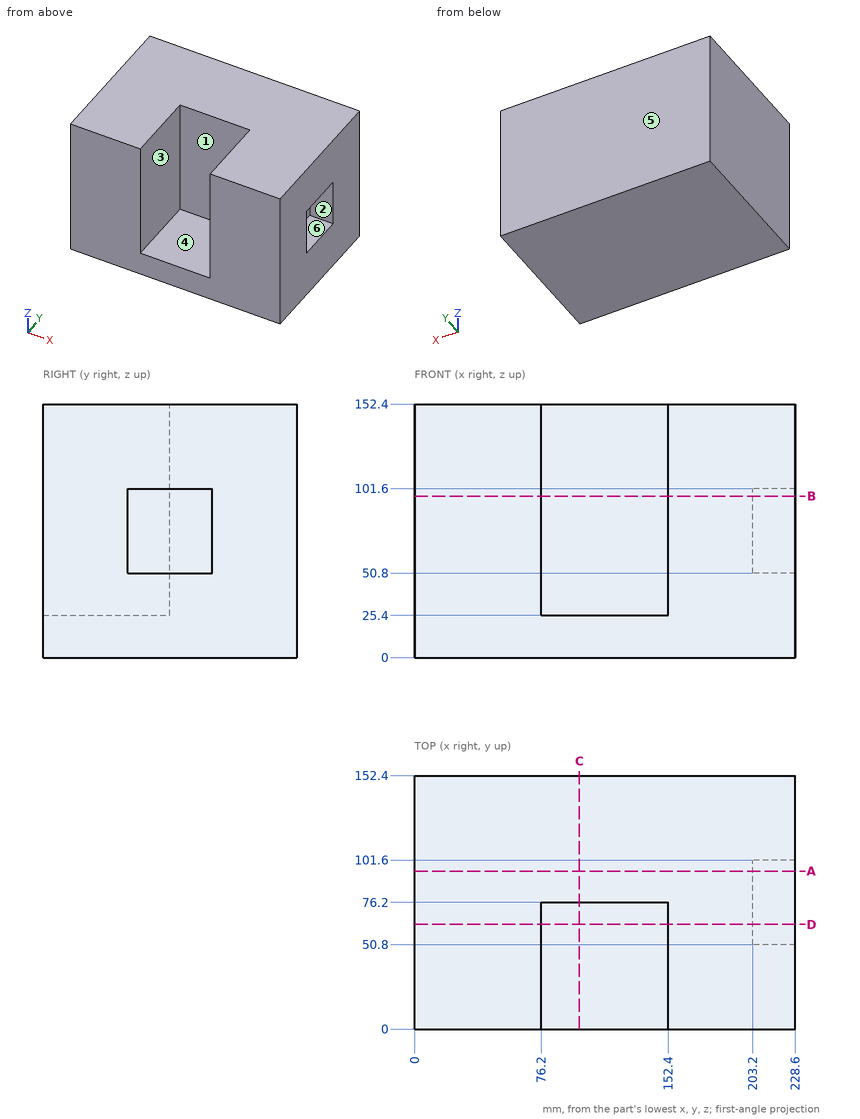
Print and shaded views of the part. All mm, measured from the part's lowest x, y and z. A direction names the side the tool comes from. Round coordinates to 2 decimals unless told otherwise and drop trailing zeros. Write each loop counter-clockwise with the first axis right and the second up, starting at its lowest first coordinate (ties: lowest second). Pieces come first, ordered by that corner, then holes. Notation, with made-up numbers: M -31.75,-33.5 L -1.75,-33.5 A26 cw -1.75,-1.5 Z; hole C 58.25,79 d11. An arc over 180 degrees is marked long. Use a Markdown table: item, result. Add a question column.
1. 3-axis set-ups, long thin cutter, end or side, ignore diameter. For the marked faces 4, 5 and 6: which of +Z, -Z, +X, -X, +Y, -Y reach the whole face in a straight line?
2. Slice it at B-B on z = 97. Give the cut face in (x, y).
3. Pull direction Y, two halves, no side cores. Call the marked faces 1, 2 and 3: released by +Y, released by -Y, zero draft, split by the parting line, or undercut.
4. Slice it at D-D on y = 63. Give the cut face in (x, z).
5. Flat gauge pins, fed straight in: P1, Ø15, axis at y = 88, z = 84, coming from the +X side; P2, Ø10, axis at x = 112.5, z = 108.5, coming from the -Y side. Where does each tip first touch, or does it go through?
6. Slice it at A-A on y = 95. Give the cut face in (x, z), then the cut area to 3 significant figures.
7. Drill centre lines: probe 1 along X at (y, z) = (63.5, 90.5); probe 2 along Y at (x, z) = (217, 93). Where is each one in solid material? Low to high.
8. Slice it at C-C on x = 99. Give the cut face in (y, z), then the cut area to 3 significant figures.
Reply:
| question | item | result |
|---|---|---|
| 1 | face 4 | +Z, -Y |
| 1 | face 5 | +Z, -Z, +X, -X, +Y |
| 1 | face 6 | +X |
| 2 | outline | M 0,0 L 76.2,0 L 76.2,76.2 L 152.4,76.2 L 152.4,0 L 228.6,0 L 228.6,50.8 L 203.2,50.8 L 203.2,101.6 L 228.6,101.6 L 228.6,152.4 L 0,152.4 Z |
| 3 | face 1 | released by -Y |
| 3 | face 2 | undercut |
| 3 | face 3 | zero draft |
| 4 | outline | M 0,0 L 228.6,0 L 228.6,50.8 L 203.2,50.8 L 203.2,101.6 L 228.6,101.6 L 228.6,152.4 L 152.4,152.4 L 152.4,25.4 L 76.2,25.4 L 76.2,152.4 L 0,152.4 Z |
| 5 | P1 | stops at x = 203.2 |
| 5 | P2 | stops at y = 76.2 |
| 6 | outline | M 0,0 L 228.6,0 L 228.6,50.8 L 203.2,50.8 L 203.2,101.6 L 228.6,101.6 L 228.6,152.4 L 0,152.4 Z |
| 6 | area | 33,500 mm^2 |
| 7 | probe 1 | x = 0 to 76.2, 152.4 to 203.2 |
| 7 | probe 2 | y = 0 to 50.8, 101.6 to 152.4 |
| 8 | outline | M 0,0 L 152.4,0 L 152.4,152.4 L 76.2,152.4 L 76.2,25.4 L 0,25.4 Z |
| 8 | area | 13,500 mm^2 |
